Read the model definition and answer for the solid it produces. Units are mm, in the model's axes. A direction names the side the tool comes from. Give positions to 0.01 mm unless a question says otherwise; leave off trailing zeros. Order: outer loops, then holes, each group sorted by start corner. A loop starts at its lowest first (then second) coordinate and runs counter-clockwise, first axis right, second up. Notation, with made-up numbers: M 18.25,16 L 69.25,16 A23 cw 69.25,34 Z; hole C -33,82 d1. An arc over 180 degrees is marked long. One line per item, written item: value. Start each with the question number.
from build123d import *

# Parameters (mm, degrees)
SKETCH1_W           = 152
SKETCH1_H           = 150
BOSS_EXTRUDE1_DEPTH = 6.5
SKETCH2_W           = 152
SKETCH2_H           = 8
BOSS_EXTRUDE2_DEPTH = 37
SKETCH3_W           = 17
SKETCH3_H           = 142
BOSS_EXTRUDE3_DEPTH = 37
SKETCH4_W           = 15
SKETCH4_H           = 142
BOSS_EXTRUDE4_DEPTH = 37
SKETCH5_W           = 120
SKETCH5_H           = 56.12
BOSS_EXTRUDE5_DEPTH = 37
HOLE2_D             = 3
HOLE2_DEPTH         = 8
HOLE2_CBORE_D       = 6
HOLE2_CBORE_DEPTH   = 4.5
HOLE3_D             = 3
HOLE3_DEPTH         = 8
HOLE3_CBORE_D       = 6
HOLE3_CBORE_DEPTH   = 4.5
HOLE4_D             = 12.5
HOLE4_DEPTH         = 17
HOLE5_D             = 3
HOLE5_CBORE_D       = 6
HOLE5_CBORE_DEPTH   = 4
HOLE6_D             = 3
HOLE6_CBORE_D       = 6
HOLE6_CBORE_DEPTH   = 4
HOLE7_D             = 3
HOLE7_CBORE_D       = 6
HOLE7_CBORE_DEPTH   = 4
HOLE9_D             = 5
HOLE9_CBORE_D       = 10
HOLE9_CBORE_DEPTH   = 23.5
HOLE10_D            = 5
HOLE10_CBORE_D      = 10
HOLE10_CBORE_DEPTH  = 23.5


with BuildPart() as part:
    # Sketch1 → Boss-Extrude1 (new body)
    with BuildSketch(Plane.XY):
        with Locations((76, 75)):
            Rectangle(SKETCH1_W, SKETCH1_H)
    extrude(amount=BOSS_EXTRUDE1_DEPTH)

    # Sketch2 → Boss-Extrude2 (add)
    with BuildSketch(Plane.XY.offset(6.5)):
        with Locations((76, 4)):
            Rectangle(SKETCH2_W, SKETCH2_H)
    extrude(amount=BOSS_EXTRUDE2_DEPTH)

    # Sketch3 → Boss-Extrude3 (add)
    with BuildSketch(Plane.XY.offset(6.5)):
        with Locations((8.5, 79)):
            Rectangle(SKETCH3_W, SKETCH3_H)
    extrude(amount=BOSS_EXTRUDE3_DEPTH)

    # Sketch4 → Boss-Extrude4 (add)
    with BuildSketch(Plane.XY.offset(6.5)):
        with Locations((144.5, 79)):
            Rectangle(SKETCH4_W, SKETCH4_H)
    extrude(amount=BOSS_EXTRUDE4_DEPTH)

    # Sketch5 → Boss-Extrude5 (add)
    with BuildSketch(Plane.XY.offset(6.5)):
        with Locations((77, 121.94)):
            Rectangle(SKETCH5_W, SKETCH5_H)
    extrude(amount=BOSS_EXTRUDE5_DEPTH)

    # Hole2
    with Locations(Plane(origin=(36.75, 0, 25.75), x_dir=(0, 0, -1), z_dir=(0, -1, 0))):
        with Locations((0, 0)):
            CounterBoreHole(HOLE2_D / 2, HOLE2_CBORE_D / 2, HOLE2_CBORE_DEPTH, depth=HOLE2_DEPTH)

    # Hole3
    with Locations(Plane(origin=(124.25, 0, 19.75), x_dir=(0, 0, -1), z_dir=(0, -1, 0))):
        with Locations((0, 0)):
            CounterBoreHole(HOLE3_D / 2, HOLE3_CBORE_D / 2, HOLE3_CBORE_DEPTH, depth=HOLE3_DEPTH)

    # Hole4
    with Locations(Plane(origin=(17, 58, 24), x_dir=(0, 1, 0), z_dir=(1, 0, 0))):
        with Locations((0, 0)):
            Hole(HOLE4_D / 2, depth=HOLE4_DEPTH)

    # Hole5 (through all)
    with Locations(Plane(origin=(94.25, 32.75, 0), x_dir=(-1, 0, 0), z_dir=(0, 0, -1))):
        with Locations((0, 0)):
            CounterBoreHole(HOLE5_D / 2, HOLE5_CBORE_D / 2, HOLE5_CBORE_DEPTH)

    # Hole6 (through all)
    with Locations(Plane(origin=(94.25, 60.75, 0), x_dir=(-1, 0, 0), z_dir=(0, 0, -1))):
        with Locations((0, 0)):
            CounterBoreHole(HOLE6_D / 2, HOLE6_CBORE_D / 2, HOLE6_CBORE_DEPTH)

    # Hole7 (through all)
    with Locations(Plane(origin=(59, 60.75, 0), x_dir=(-1, 0, 0), z_dir=(0, 0, -1))):
        with Locations((0, 0)):
            CounterBoreHole(HOLE7_D / 2, HOLE7_CBORE_D / 2, HOLE7_CBORE_DEPTH)

    # Hole9 (through all)
    with Locations(Plane(origin=(132, 126, 0), x_dir=(-1, 0, 0), z_dir=(0, 0, -1))):
        with Locations((0, 0), (112, 0)):
            CounterBoreHole(HOLE9_D / 2, HOLE9_CBORE_D / 2, HOLE9_CBORE_DEPTH)

    # Hole10 (through all)
    with Locations(Plane(origin=(143.5, 15, 0), x_dir=(-1, 0, 0), z_dir=(0, 0, -1))):
        with Locations((0, 0), (135, 0)):
            CounterBoreHole(HOLE10_D / 2, HOLE10_CBORE_D / 2, HOLE10_CBORE_DEPTH)


solid = part.part
Q1. Consider probe 1 along Y at (x, z) = (131.5, 9); probe 2 along Y at (x, z) = (94, 2); probe 3 along Y at (x, z) = (80, 13.5). Determine where each line is inside the solid, lowest interval first.
Q2. Find section C-C, the plane x = 143.5. Give the vertices of the cut face in (y, z).
Q3. Find section D-D, the plane x = 72.5. Give the vertices of the cut face in (y, z), then the cut area to 3 significant figures.
Q4. A tool of negligible diameter and unlimited length cuts with its end or side. For faces 5 (the flat face through (76, 8, 25)), 6 (the flat face through (96, 32, 4)), 7 (the cylindrical face through (38.78, 2.22, 27.96)), 8 (the cylindrical face through (10, 13, 34)), from which of +Z, -Z, +X, -X, +Y, -Y can it reach the whole face along a straight path? Write none if from no direction.
Q5. Find section B-B, the plane z = 8.5. Give the vertices of the cut face in (x, y), then the cut area to 3 significant figures.
Q6. Find section A-A, the plane y = 15. Give the vertices of the cut face in (x, z), then the cut area to 3 significant figures.
Q7. Determine the mould class of faces 1 (the flat face through (75, 109, 43.5)), 2 (the flat face through (35, 4.5, 24)), 3 (the cylindrical face through (8.38, 52.04, 25.88)), 4 (the cylindrical face through (97.247, 32.882, 1.972)) for opening direction Z: released by +Z, released by -Z, zero draft, split by the parting line, or undercut.
Q8. Each of these flat-tipped pins is pushed along its axis until it touches: pin 1 (3 mm diameter, centred on x = 77.5, y = 37.5, fed in from +Z); pin 2 (8 mm diameter, centred on x = 143, y = 15.5, fed in from -Z); pin 3 (3.5 mm diameter, centred on x = 94.25, y = 60.75, fed in from -Z). Where does it stop, or does it pass through?
Evaluation:
1. probe 1: 0 to 8, 93.88 to 121.03, 130.97 to 150
1. probe 2: 0 to 29.76, 35.74 to 57.76, 63.74 to 150
1. probe 3: 0 to 8, 93.88 to 150
2. outline: M 0,0 L 10,0 L 10,23.5 L 12.5,23.5 L 12.5,43.5 L 0,43.5 Z; M 17.5,23.5 L 20,23.5 L 20,0 L 150,0 L 150,43.5 L 17.5,43.5 Z
3. outline: M 0,0 L 150,0 L 150,43.5 L 93.88,43.5 L 93.88,6.5 L 8,6.5 L 8,43.5 L 0,43.5 Z
3. area: 3,350 mm2
4. face 5: +Z
4. face 6: -Z
4. face 7: -Y
4. face 8: +Z, -Z
5. outline: M 0,0 L 152,0 L 152,150 L 0,150 Z; hole C 8.5,15 d10; hole C 20,126 d10; hole M 17,8 L 137,8 L 137,93.88 L 17,93.88 Z; hole C 132,126 d10; hole C 143.5,15 d10
5. area: 12,200 mm2
6. outline: M 0,0 L 3.5,0 L 3.5,23.5 L 6,23.5 L 6,43.5 L 0,43.5 Z; M 11,23.5 L 13.5,23.5 L 13.5,0 L 138.5,0 L 138.5,23.5 L 141,23.5 L 141,43.5 L 137,43.5 L 137,6.5 L 17,6.5 L 17,43.5 L 11,43.5 Z; M 146,23.5 L 148.5,23.5 L 148.5,0 L 152,0 L 152,43.5 L 146,43.5 Z
6. area: 1,500 mm2
7. face 1: released by +Z
7. face 2: undercut
7. face 3: undercut
7. face 4: zero draft
8. pin 1: z = 6.5
8. pin 2: z = 23.5
8. pin 3: z = 4
